```python
from build123d import *

# Parameters (mm, degrees)
F1_DEPTH      = 2
F1_DEPTH_BACK = 2


with BuildPart() as f1:
    # F0 (on Right) → F1 (new body, two sides)
    with BuildSketch(Plane.YZ) as f1_sk:
        with BuildLine():
            Line((0, 100), (0, 0))
            Line((0, 0), (73.031177, -200.651511))
            ThreePointArc((73.031177, -200.651511), (100.489891, -236.436403), (143.508124, -250))
            Line((143.508124, -250), (425, -250))
            ThreePointArc((425, -250), (442.67767, -242.67767), (450, -225))
            Line((450, -225), (450, 0))
            Line((450, 0), (450, 225))
            ThreePointArc((450, 225), (442.67767, 242.67767), (425, 250))
            Line((425, 250), (380, 250))
            ThreePointArc((380, 250), (362.32233, 242.67767), (355, 225))
            Line((355, 225), (355, 35))
            Line((355, 35), (35, 35))
            Line((35, 35), (35, 100))
            Line((35, 100), (0, 100))
        make_face()
    extrude(amount=F1_DEPTH)
    extrude(f1_sk.sketch, amount=-F1_DEPTH_BACK)


solid = f1.part
```
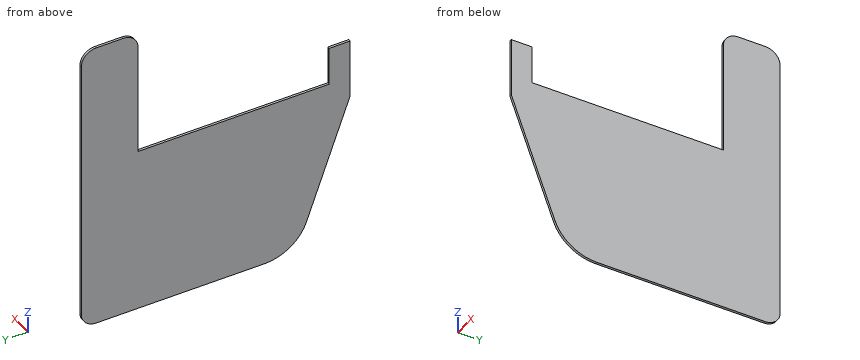
The listing builds one solid part. Answer for the finished solid, in the listing's coordinates (mm). Coordinates: 2 decimals unless noted, no trailing zeros. Loops run counter-clockwise (first coordinate to the right, second up) from the corner with the lowest first, then second, coordinate; pieces in that order, holes last. Notation, with made-up numbers: (-15, 45.5) - (43, 45.5) arc R29 cw to (43, 67.5) - close; hole circle Ø11 at (15, 50). An arc over 180 degrees is marked (long way). Use a Markdown table: item, result. Add a question column.
1) Given pin 1 (1.2 mm diameter, centred on x = 1, y = 10, fed in from +Z); pin 2 (1.2 mm diameter, centred on x = 0.5, z = 152, fed in from -Y); pin 3 (1.2 mm diameter, centred on x = 0, y = 216.5, fed in from +Z), each flat-ended and moving along its own axis, determine where each tip first touches the part or whether it passes through.
2) The part is cut by section B-B, the plane x = 0.3. Give the vertices of the cut face in (y, z), and give its area (3 significant figures).
3) The part is cut by section C-C, the plane y = 202.5. Give the vertices of the cut face in (x, z), and give its area (3 significant figures).
4) The part is cut by section A-A, the plane z = 71.5. Give the vertices of the cut face in (x, y).
5) Find the intervals of material crossed by line 1 (Y direction, x = 1.75, z = 36); line 2 (Y direction, x = 1.4, z = 105); line 3 (Z direction, x = -1.7, y = 280), in increasing order.
6) The part is cut by section D-D, the plane z = 214.5. Give the vertices of the cut face in (x, y), and give its area (3 significant figures).
Here are the results:
| question | item | result |
|---|---|---|
| 1 | pin 1 | stops at z = 100 |
| 1 | pin 2 | stops at y = 355 |
| 1 | pin 3 | stops at z = 35 |
| 2 | outline | (0, 0) - (73.03, -200.65) arc R75 ccw to (143.51, -250) - (425, -250) arc R25 ccw to (450, -225) - (450, 225) arc R25 ccw to (425, 250) - (380, 250) arc R25 ccw to (355, 225) - (355, 35) - (35, 35) - (35, 100) - (0, 100) - close |
| 2 | area | 139,000 mm^2 |
| 3 | outline | (-2, -250) - (2, -250) - (2, 35) - (-2, 35) - close |
| 3 | area | 1,140 mm^2 |
| 4 | outline | (-2, 0) - (2, 0) - (2, 35) - (-2, 35) - close; (-2, 355) - (2, 355) - (2, 450) - (-2, 450) - close |
| 5 | line 1 | y = 0 to 35, 355 to 450 |
| 5 | line 2 | y = 355 to 450 |
| 5 | line 3 | z = -250 to 35 |
| 6 | outline | (-2, 355) - (2, 355) - (2, 450) - (-2, 450) - close |
| 6 | area | 380 mm^2 |
